Study the drawing (mm; zero at the part's minimum x, y, z) and answer. Coordinates: 2 decimals unless noted, no trailing zeros. Write each question's results on one line, items separated by ' | '. Start each with the question number.
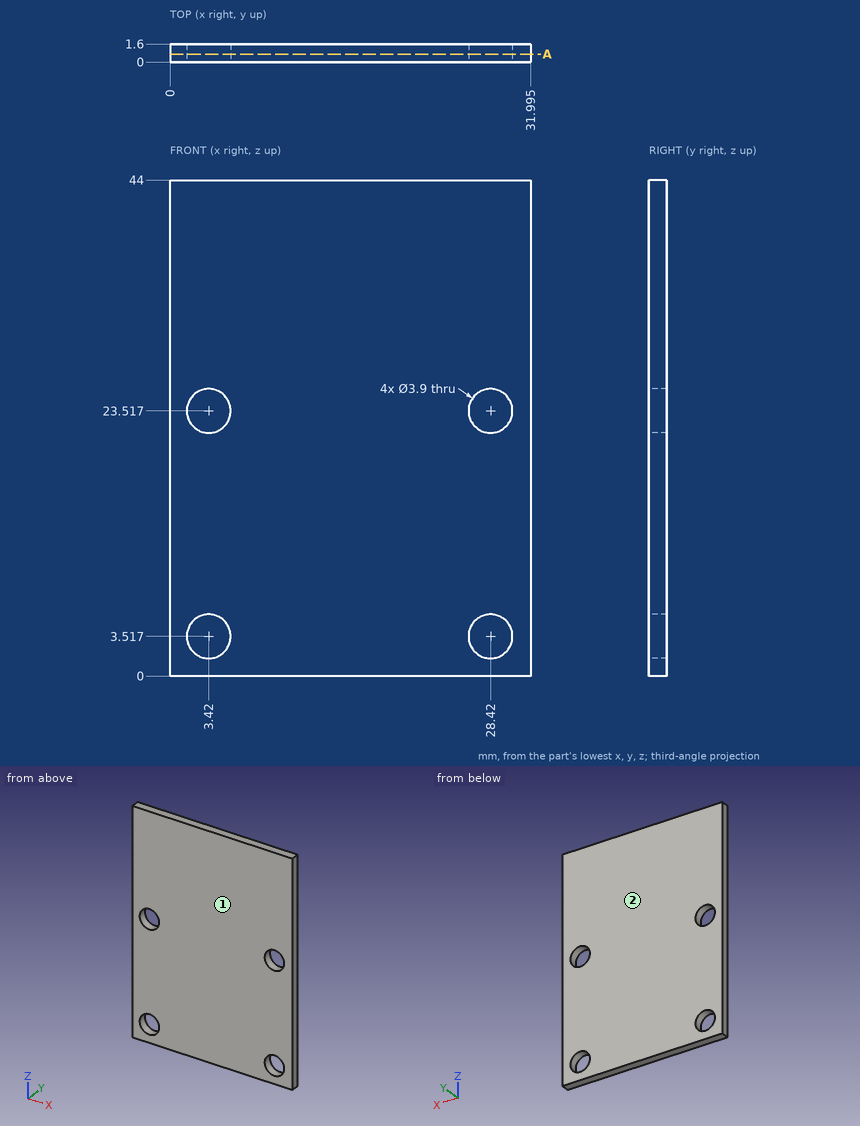
1. Determine the mould class of the marked faces 1 and 2 for opening direction Y: pulls with the +Y half, pulls with the -Y half, needs draft (parallel to the pull), parting line crosses it, or undercut.
2. Given pin 1 Ø3 at (x, z) = (3.42, 23.52) entering from +Y, flat-ended and moving along its own axis, determine where the tip first touches the part or whether it passes through.
3. Find section A-A on y = 0.7. Give the number of separate pieces and of enclosed holes in the cut face, and give its area (3 significant figures).
4. Find the intervals of material crossed by L1, parallel to Z at x = 27.5, y = 0.75 (1 decimal); L2, parallel to Z at x = 28, y = 0.95; L3, parallel to X at y = 1.35, z = 24 (1 decimal), in increasing order.
Ans:
1) face 1: pulls with the -Y half | face 2: pulls with the +Y half
2) pin 1: passes through
3) separate pieces: 1 | enclosed holes: 4 | area: 1,360 mm²
4) L1: z = 0 to 1.8, 5.2 to 21.8, 25.2 to 44 | L2: z = 0 to 1.61, 5.42 to 21.61, 25.42 to 44 | L3: x = 0 to 1.5, 5.3 to 26.5, 30.3 to 32
